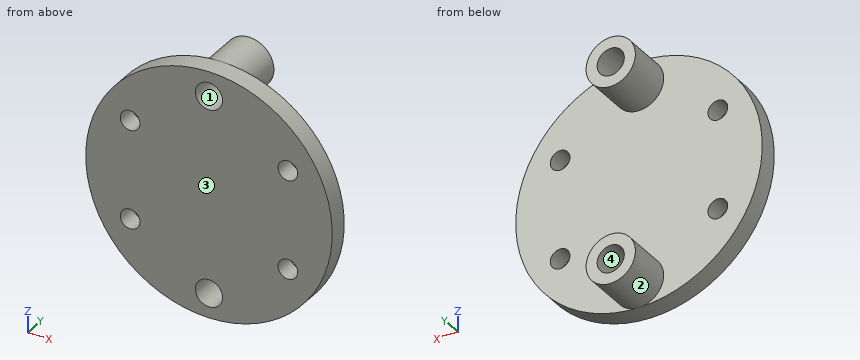
```python
from build123d import *

# Parameters (mm, degrees)
SKETCH1_R           = 15.875
SKETCH1_R_2         = 1.75
SKETCH1_W           = 25.4
SKETCH1_H           = 17.78
SKETCH1_R_3         = 1.27
BOSS_EXTRUDE1_DEPTH = 2.54
SKETCH2_R           = 3.175
SKETCH2_R_2         = 1.75
BOSS_EXTRUDE2_DEPTH = 5.974999988


with BuildPart() as part:
    # Sketch1 → Boss-Extrude1 (new body)
    # profile 1 of 2: a face of its own
    with BuildSketch(Plane(origin=(0, 0, 0), x_dir=(1, 0, 0), z_dir=(0, 1, 0))):
        with Locations(Location((12.7, 8.89, 0), (0, 0, 270))):
            Circle(SKETCH1_R)
        with Locations(Location((12.7, 21.59, 0), (0, 0, 270))):
            Circle(SKETCH1_R_2, mode=Mode.SUBTRACT)
        with Locations(Location((12.7, -3.81, 0), (0, 0, 270))):
            Circle(SKETCH1_R_2, mode=Mode.SUBTRACT)
        with Locations((12.7, 8.89)):
            Rectangle(SKETCH1_W, SKETCH1_H, mode=Mode.SUBTRACT)
    # profile 2 of 2: a face of its own
    with BuildSketch(Plane(origin=(0, 0, 0), x_dir=(1, 0, 0), z_dir=(0, 1, 0))):
        with Locations((12.7, 8.89)):
            Rectangle(SKETCH1_W, SKETCH1_H)
        with Locations(Location((22.86, 15.24, 0), (0, 0, 270))):
            Circle(SKETCH1_R_3, mode=Mode.SUBTRACT)
        with Locations(Location((2.54, 15.24, 0), (0, 0, 270))):
            Circle(SKETCH1_R_3, mode=Mode.SUBTRACT)
        with Locations(Location((22.86, 2.54, 0), (0, 0, 270))):
            Circle(SKETCH1_R_3, mode=Mode.SUBTRACT)
        with Locations(Location((2.54, 2.54, 0), (0, 0, 270))):
            Circle(SKETCH1_R_3, mode=Mode.SUBTRACT)
    extrude(amount=BOSS_EXTRUDE1_DEPTH)

    # Sketch2 → Boss-Extrude2 (add)
    # profile 1 of 2: a face of its own
    with BuildSketch(Plane(origin=(0, 2.54, 0), x_dir=(1, 0, 0), z_dir=(0, 1, 0))):
        with Locations(Location((12.7, 21.59, 0), (0, 0, 89.999491582))):
            Circle(SKETCH2_R)
        with Locations(Location((12.7, 21.59, 0), (0, 0, 270))):
            Circle(SKETCH2_R_2, mode=Mode.SUBTRACT)
    # profile 2 of 2: a face of its own
    with BuildSketch(Plane(origin=(0, 2.54, 0), x_dir=(1, 0, 0), z_dir=(0, 1, 0))):
        with Locations(Location((12.7, -3.81, 0), (0, 0, 269.999491581))):
            Circle(SKETCH2_R)
        with Locations(Location((12.7, -3.81, 0), (0, 0, 270))):
            Circle(SKETCH2_R_2, mode=Mode.SUBTRACT)
    extrude(amount=BOSS_EXTRUDE2_DEPTH)


solid = part.part
```
Could you check a few things on this model? Use its own coordinates, in mm. Face numbers are marked on the shaded views. A direction names the side the tool comes from. Give positions to 0.01 mm unless a question says otherwise; leave off trailing zeros. Loops run counter-clockwise (first coordinate to the right, second up) from the corner with the lowest first, then second, coordinate; pieces in that order, holes last. Notation, with made-up numbers: (-25.75, -2) -> (-7.75, -2) arc R16 ccw to (-7.75, 26) -> close; hole circle Ø4 at (16, -3.5). An arc over 180 degrees is marked (long way). Put each result on its own line as item: value.
(1) Imagine slicing it at A-A on x = 3. Write out the boundary of the cut face in (y, z).
Computed:
outline: (0, -21.46) -> (2.54, -21.46) -> (2.54, -16.42) -> (0, -16.42) -> close; (0, -14.06) -> (2.54, -14.06) -> (2.54, -3.72) -> (0, -3.72) -> close; (0, -1.36) -> (2.54, -1.36) -> (2.54, 3.68) -> (0, 3.68) -> close
(2) Imagine slicing it at D-D on y = 6. Write out the boundary of the cut face in (x, z) (3 decimals).
Computed:
outline: circle Ø6.35 at (12.7, -21.59); circle Ø6.35 at (12.7, 3.81); hole circle Ø3.5 at (12.7, -21.59); hole circle Ø3.5 at (12.7, 3.81)
(3) Thinking about a two-plate mould opening in Z: for the marked faces 3 and 4, which applies, pulls with the +Z half, pulls with the -Z half, needs draft (parallel to the pull), parting line crosses it, or undercut?
Computed:
face 3: needs draft
face 4: undercut
(4) For the marked faces 1 and 2, which set-ups out of +Z, -Z, +X, -X, +Y, -Y let a thin tool reach every point of the face, with its end or its side?
Computed:
face 1: +Y, -Y
face 2: +Y
(5) I'm going to push flat-ended pins straight in: pin 1 Ø1.5 at (y, z) = (7.5, -18) entering from +X; pin 2 Ø4 at (x, z) = (2.54, -15.24) entering from +Y; pin 3 Ø1.5 at (x, z) = (2.54, -2.54) entering from -Y; pin 4 Ø5 at (y, z) = (3, -12) entering from -X. Where does each tip first touch, or does it pass through?
Computed:
pin 1: x = 14.12
pin 2: y = 2.54
pin 3: through
pin 4: x = -3.16
(6) Please list where these lines run through material, in increasing order: probe 1 along X at (y, z) = (1.9, -15.24); probe 2 along X at (y, z) = (6.25, 3.81) (3 decimals); probe 3 along Y at (x, z) = (15, -7.5). Write a range as [from, to].
Computed:
probe 1: [-1.85, 1.27], [3.81, 21.59], [24.13, 27.25]
probe 2: [9.525, 10.95], [14.45, 15.875]
probe 3: [0, 2.54]
(7) Imagine slicing it at C-C on z = -2.54. Write out the boundary of the cut face in (x, y), plus the area to 3 significant figures.
Computed:
outline: (-1.85, 0) -> (1.27, 0) -> (1.27, 2.54) -> (-1.85, 2.54) -> close; (3.81, 0) -> (21.59, 0) -> (21.59, 2.54) -> (3.81, 2.54) -> close; (24.13, 0) -> (27.25, 0) -> (27.25, 2.54) -> (24.13, 2.54) -> close
area: 61.0 mm^2
(8) Imagine slicing it at B-B on y = 1.75. Write out the boundary of the cut face in (x, z) (3 decimals), plus the area to 3 significant figures.
Computed:
outline: circle Ø31.75 at (12.7, -8.89); hole circle Ø2.54 at (2.54, -15.24); hole circle Ø2.54 at (2.54, -2.54); hole circle Ø3.5 at (12.7, -21.59); hole circle Ø3.5 at (12.7, 3.81); hole circle Ø2.54 at (22.86, -15.24); hole circle Ø2.54 at (22.86, -2.54)
area: 752 mm^2
